Design review of the part shown in the three views and the two pictorial views. Dimensions are in mm from the part's minimum x, y and z. Coordinates: 2 decimals unless noted, no trailing zeros. Loops run counter-clockwise (first coordinate to the right, second up) from the corner with the lowest first, then second, coordinate; pieces in that order, holes last. Notation, with made-up numbers: M -20,-29 L 28,-29 A5 ccw 28,-25 Z; hole C -28,38.5 d9. An arc over 180 degrees is marked long. Use CSV: the item, a comma, the result in double quotes. Start each with the question number.
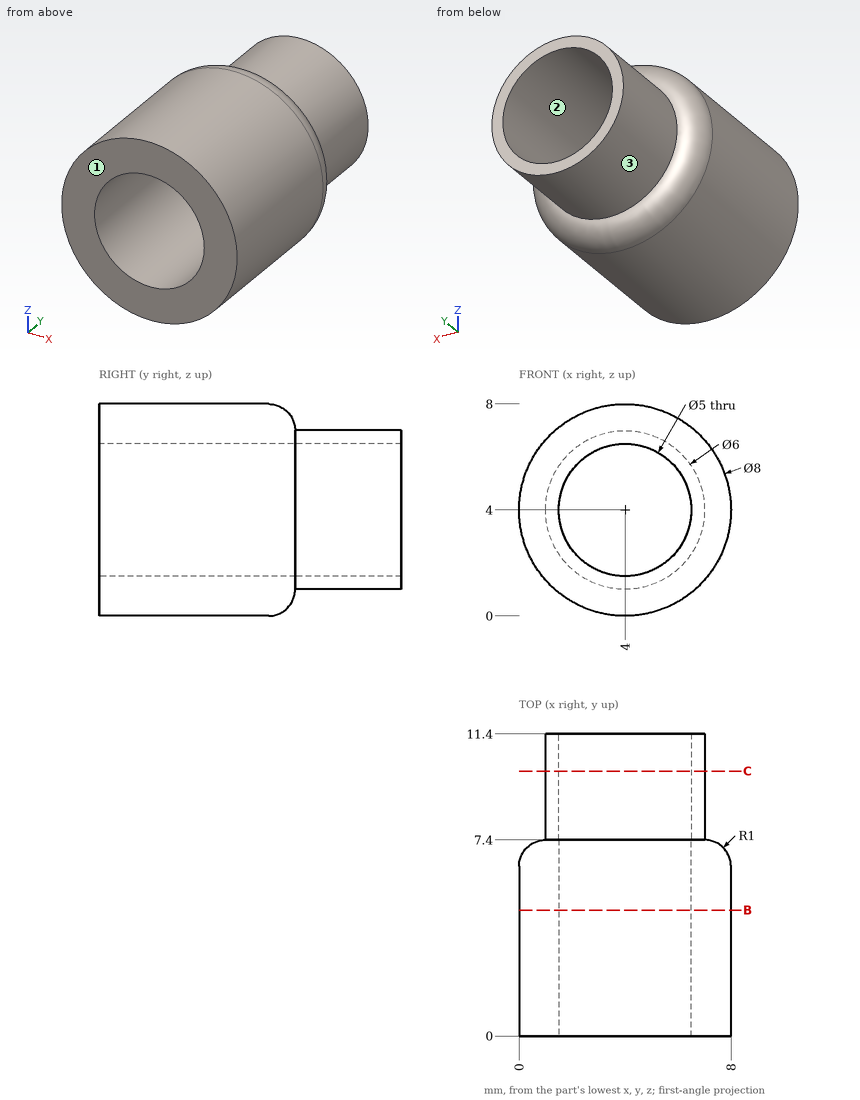
1. Draft analysis for pull direction Z (two halves, no side actions). For the marked faces 1, 2 and 3, state which applies: released by +Z, released by -Z, zero draft, split by the parting line, or undercut.
2. To check wall thickness, follow line 1 along X through (y, z) = (3.5, 4); line 2 along Z through (x, y) = (4, 8.75); line 3 along Z through (x, y) = (2, 6.5). State the ranges of each line that lie inside material, in increasing order.
3. Insertion check: pin 1 Ø2 at (y, z) = (6.5, 2) entering from +X. The pin has a flat end and moves straight along its axis. Give the tip position at first contact, or say it passes through.
4. Add section C-C (y = 10). Write out the cut boundary in (x, z).
5. Add section B-B (y = 4.75). Write out the cut boundary in (x, z), plus the area to 3 significant figures.
Solved:
1,face 1,"zero draft"
1,face 2,"undercut"
1,face 3,"split by the parting line"
2,line 1,"x = 0 to 1.5, 6.5 to 8"
2,line 2,"z = 1 to 1.5, 6.5 to 7"
2,line 3,"z = 0.54 to 2.5, 5.5 to 7.46"
3,pin 1,"stops at x = 7.87"
4,outline,"C 4,4 d6; hole C 4,4 d5"
5,outline,"C 4,4 d8; hole C 4,4 d5"
5,area,"30.6 mm^2"
